The listing builds one solid part. Answer for the finished solid, in the listing's coordinates (mm). A direction names the side the tool comes from. Coordinates: 2 decimals unless noted, no trailing zeros. Order: outer loops, then holes, each group sorted by start corner. A loop starts at its lowest first (then second) coordinate and runs counter-clockwise, first axis right, second up. Notation, with made-up numbers: (30.5, 56) -> (34.5, 56) arc R10 ccw to (34.5, 71) -> close; hole circle Ø9 at (-40, 71.25). An arc over 180 degrees is marked (long way). Write item = value, one per line. Start each with the question number.
```python
from build123d import *

# Parameters (mm, degrees)
SKETCH1_R           = 75
SKETCH1_R_2         = 7.5
BOSS_EXTRUDE1_DEPTH = 10
SKETCH2_R           = 7.5
BOSS_EXTRUDE2_DEPTH = 30
SKETCH3_R           = 75
SKETCH3_R_2         = 7.5
BOSS_EXTRUDE5_DEPTH = 10


with BuildPart() as part:
    # Sketch1 → Boss-Extrude1 (new body)
    with BuildSketch(Plane(origin=(0, 0, 0), x_dir=(1, 0, 0), z_dir=(0, 1, 0))):
        with Locations(Location((0, 0, 0), (0, 0, 270))):
            Circle(SKETCH1_R)
        with Locations(Location((60, 0, 0), (0, 0, 270))):
            Circle(SKETCH1_R_2, mode=Mode.SUBTRACT)
    extrude(amount=BOSS_EXTRUDE1_DEPTH)

    # Sketch2 → Boss-Extrude2 (add)
    with BuildSketch(Plane(origin=(0, 10, 0), x_dir=(1, 0, 0), z_dir=(0, 1, 0))):
        with Locations(Location((0, 0, 0), (0, 0, 270))):
            Circle(SKETCH2_R)
    extrude(amount=BOSS_EXTRUDE2_DEPTH)

    # Sketch3 → Boss-Extrude5 (add)
    with BuildSketch(Plane(origin=(0, 40, 0), x_dir=(1, 0, 0), z_dir=(0, 1, 0))):
        with Locations(Location((0, 0, 0), (0, 0, 270))):
            Circle(SKETCH3_R)
        with Locations(Location((59.088465181, 10.41889066, 0), (0, 0, 270))):
            Circle(SKETCH3_R_2, mode=Mode.SUBTRACT)
    extrude(amount=BOSS_EXTRUDE5_DEPTH)


solid = part.part
```
Item 1: Section A-A, the plane z = 0 is taken. Give the vertices of the cut face in (x, y).
Item 2: Section B-B, the plane x = -56 is taken. Give the vertices of the cut face in (y, z), then the cut area to 3 significant figures.
Item 3: Section C-C, the plane z = 62.5 is taken. Give the vertices of the cut face in (x, y), then the cut area to 3 significant figures.
Item 4: Section D-D, the plane x = 0 is taken. Give the vertices of the cut face in (y, z).
Item 5: Consider probe 1 along Y at (x, z) = (15, -9); probe 2 along Z at (x, y) = (-18, 7.5); probe 3 along Z at (x, y) = (43, 6.5). Determine where each line is inside the solid, lowest interval first.
Item 6: Each of these flat-tipped pins is pushed along its axis until it touches: pin 1 (8 mm diameter, centred on y = 14.5, z = 55, fed in from -X); pin 2 (8 mm diameter, centred on x = -6, y = 35, fed in from -Z); pin 3 (1.5 mm diameter, centred on y = 42, z = 22.5, fed in from -X); pin 4 (12 mm diameter, centred on x = 60, z = 0, fed in from -Y). Where does it stop, or does it pass through?
Item 7: For a pull along Y with two mould halves and no side action, classify faces 3 (the flat face through (1, 50, -1)), 4 (the flat face through (1, 0, -1)), 5 (the cylindrical face through (67.436, 4.93, -0.976)), 6 (the cylindrical face through (0.33, 24.79, -7.493)) as pulls with the +Y half, pulls with the -Y half, needs draft (parallel to the pull), parting line crosses it, or undercut.
Item 8: Which of the six approach directions +Z, -Z, +X, -X, +Y, -Y give full straight-line access (tool end or side, diameter ignored) to faces 1 (the cylindrical face through (-45.636, 44.93, -59.517)), 2 (the cylindrical face through (66.525, 44.93, -11.395))?
A:
q1.outline = (-75, 0) -> (52.5, 0) -> (52.5, 10) -> (7.5, 10) -> (7.5, 40) -> (75, 40) -> (75, 50) -> (-75, 50) -> (-75, 40) -> (-7.5, 40) -> (-7.5, 10) -> (-75, 10) -> close; (67.5, 0) -> (75, 0) -> (75, 10) -> (67.5, 10) -> close
q2.outline = (0, -49.89) -> (10, -49.89) -> (10, 49.89) -> (0, 49.89) -> close; (40, -49.89) -> (50, -49.89) -> (50, 49.89) -> (40, 49.89) -> close
q2.area = 2,000 mm^2
q3.outline = (-41.46, 0) -> (41.46, 0) -> (41.46, 10) -> (-41.46, 10) -> close; (-41.46, 40) -> (41.46, 40) -> (41.46, 50) -> (-41.46, 50) -> close
q3.area = 1,660 mm^2
q4.outline = (0, -75) -> (10, -75) -> (10, -7.5) -> (40, -7.5) -> (40, -75) -> (50, -75) -> (50, 75) -> (40, 75) -> (40, 7.5) -> (10, 7.5) -> (10, 75) -> (0, 75) -> close
q5.probe_1 = 0 to 10, 40 to 50
q5.probe_2 = -72.81 to 72.81
q5.probe_3 = -61.45 to 61.45
q6.pin_1 = through
q6.pin_2 = -7.23
q6.pin_3 = -71.78
q6.pin_4 = 40
q7.face_3 = pulls with the +Y half
q7.face_4 = pulls with the -Y half
q7.face_5 = needs draft
q7.face_6 = undercut
q8.face_1 = +Y, -Y
q8.face_2 = +Y
